from build123d import *

# Parameters (mm, degrees)
SKETCH_1_R          = 25
SKETCH_1_R_2        = 8
SKETCH_1_R_3        = 1.65
EXTRUDE_1_DEPTH     = 4
SKETCH_5_W          = 23.4
SKETCH_5_H          = 29.4
CUT_EXTRUDE_1_DEPTH = 1
SKETCH_6_R          = 3
CUT_EXTRUDE_2_DEPTH = 2.8
CUT_EXTRUDE_3_REACH = 37.482
SKETCH_9_R          = 0.75
CUT_EXTRUDE_START   = -1.1
CUT_EXTRUDE_4_DEPTH = 1.1


with BuildPart() as part:
    # 草图1 → 凸台-拉伸1 (new body)
    with BuildSketch(Plane(origin=(0, 0, 0), x_dir=(1, 0, 0), z_dir=(0, 1, 0))):
        with Locations(Location((0, 0, 0), (0, 0, 270))):
            Circle(SKETCH_1_R)
        with Locations(Location((0, 0, 0), (0, 0, 270))):
            Circle(SKETCH_1_R_2, mode=Mode.SUBTRACT)
        with Locations(Location((10.606601718, 10.606601718, 0), (0, 0, 270))):
            Circle(SKETCH_1_R_3, mode=Mode.SUBTRACT)
        with Locations(Location((-10.606601718, 10.606601718, 0), (0, 0, 270))):
            Circle(SKETCH_1_R_3, mode=Mode.SUBTRACT)
        with Locations(Location((-10.606601718, -10.606601718, 0), (0, 0, 270))):
            Circle(SKETCH_1_R_3, mode=Mode.SUBTRACT)
        with Locations(Location((10.606601718, -10.606601718, 0), (0, 0, 270))):
            Circle(SKETCH_1_R_3, mode=Mode.SUBTRACT)
    extrude(amount=EXTRUDE_1_DEPTH)

    # 草图5 → 切除-拉伸1 (cut)
    with BuildSketch(Plane(origin=(0, 4, 0), x_dir=(1, 0, 0), z_dir=(0, 1, 0))):
        with Locations((0, 6)):
            Rectangle(SKETCH_5_W, SKETCH_5_H)
    extrude(amount=-CUT_EXTRUDE_1_DEPTH, mode=Mode.SUBTRACT)

    # 草图6 → 切除-拉伸2 (cut)
    with BuildSketch(Plane(origin=(0, 4, 0), x_dir=(1, 0, 0), z_dir=(0, 1, 0))):
        with Locations(Location((-10.606601718, 10.606601718, 0), (0, 0, 270))):
            Circle(SKETCH_6_R)
        with Locations(Location((10.606601718, 10.606601718, 0), (0, 0, 270))):
            Circle(SKETCH_6_R)
        with Locations(Location((10.606601718, -10.606601718, 0), (0, 0, 270))):
            Circle(SKETCH_6_R)
        with Locations(Location((-10.606601718, -10.606601718, 0), (0, 0, 270))):
            Circle(SKETCH_6_R)
    extrude(amount=-CUT_EXTRUDE_2_DEPTH, mode=Mode.SUBTRACT)

    # 草图9 → 切除-拉伸3 (cut, up to next)
    with BuildSketch(Plane(origin=(0, 3, 0), x_dir=(1, 0, 0), z_dir=(0, 1, 0)), mode=Mode.PRIVATE) as cut_extrude_3_sk1:
        with Locations(Location((-8.5, 5.5, 0), (0, 0, 270))):
            Circle(SKETCH_9_R)
    cut_extrude_3_tool1 = extrude(cut_extrude_3_sk1.sketch, amount=-CUT_EXTRUDE_3_REACH, mode=Mode.PRIVATE) & part.part
    # 草图9 → 切除-拉伸3 (cut, up to next)
    with BuildSketch(Plane(origin=(0, 3, 0), x_dir=(1, 0, 0), z_dir=(0, 1, 0)), mode=Mode.PRIVATE) as cut_extrude_3_sk2:
        with Locations(Location((8.5, 5.5, 0), (0, 0, 270))):
            Circle(SKETCH_9_R)
    cut_extrude_3_tool2 = extrude(cut_extrude_3_sk2.sketch, amount=-CUT_EXTRUDE_3_REACH, mode=Mode.PRIVATE) & part.part
    # 草图9 → 切除-拉伸3 (cut, up to next)
    with BuildSketch(Plane(origin=(0, 3, 0), x_dir=(1, 0, 0), z_dir=(0, 1, 0)), mode=Mode.PRIVATE) as cut_extrude_3_sk3:
        with Locations(Location((8.5, -5.5, 0), (0, 0, 270))):
            Circle(SKETCH_9_R)
    cut_extrude_3_tool3 = extrude(cut_extrude_3_sk3.sketch, amount=-CUT_EXTRUDE_3_REACH, mode=Mode.PRIVATE) & part.part
    # 草图9 → 切除-拉伸3 (cut, up to next)
    with BuildSketch(Plane(origin=(0, 3, 0), x_dir=(1, 0, 0), z_dir=(0, 1, 0)), mode=Mode.PRIVATE) as cut_extrude_3_sk4:
        with Locations(Location((-8.5, -5.5, 0), (0, 0, 270))):
            Circle(SKETCH_9_R)
    cut_extrude_3_tool4 = extrude(cut_extrude_3_sk4.sketch, amount=-CUT_EXTRUDE_3_REACH, mode=Mode.PRIVATE) & part.part
    add(cut_extrude_3_tool1.solids().sort_by_distance((-8.5, 3, -5.5))[0], mode=Mode.SUBTRACT)
    add(cut_extrude_3_tool2.solids().sort_by_distance((8.5, 3, -5.5))[0], mode=Mode.SUBTRACT)
    add(cut_extrude_3_tool3.solids().sort_by_distance((8.5, 3, 5.5))[0], mode=Mode.SUBTRACT)
    add(cut_extrude_3_tool4.solids().sort_by_distance((-8.5, 3, 5.5))[0], mode=Mode.SUBTRACT)

    # 草图10 → 切除-拉伸4 (cut)
    with BuildSketch(Plane(origin=(0, 3, 0), x_dir=(1, 0, 0), z_dir=(0, 1, 0)).offset(CUT_EXTRUDE_START)):
        with BuildLine():
            Line((-5.700788223, 5.612576381), (-5.700788223, 6.246626792))
            ThreePointArc((-5.700788223, 6.246626792), (-5.993681442, 6.953733574), (-6.700788223, 7.246626792))
            Line((-6.700788223, 7.246626792), (-11.441421376, 7.246626792))
            Line((-11.441421376, 7.246626792), (-11.441421376, 20.219080974))
            Line((-11.441421376, 20.219080974), (11.441421376, 20.219080974))
            Line((11.441421376, 20.219080974), (11.441421376, 7.246626792))
            Line((11.441421376, 7.246626792), (6.700788223, 7.246626792))
            ThreePointArc((6.700788223, 7.246626792), (5.993681442, 6.953733574), (5.700788223, 6.246626792))
            Line((5.700788223, 6.246626792), (5.700788223, 5.612576381))
            ThreePointArc((5.700788223, 5.612576381), (0, 8), (-5.700788223, 5.612576381))
        make_face()
    extrude(amount=CUT_EXTRUDE_4_DEPTH, mode=Mode.SUBTRACT)


solid = part.part
Design review of the part built by this model. Coordinates are the model's own, in mm. A direction names the side the tool comes from. Coordinates: 2 decimals unless noted, no trailing zeros. Order: outer loops, then holes, each group sorted by start corner. A loop starts at its lowest first (then second) coordinate and runs counter-clockwise, first axis right, second up. Notation, with made-up numbers: (10, 19) - (34, 19) arc R18 ccw to (34, 42) - close; hole circle Ø9 at (87, 23). An arc over 180 degrees is marked (long way). Put each result on its own line as item: value.
1) Insertion check: P1, Ø16, axis at x = 2, z = -10.5, coming from the +Y side; P2, Ø1.1, axis at y = 3.5, z = -3, coming from the -X side; P3, Ø3, axis at x = -10.5, z = 9.5, coming from the +Y side. Each pin has a flat end and moves straight along its axis. Give the tip position at first contact, or say it passes through.
Response values:
P1: stops at y = 3
P2: stops at x = -24.88
P3: stops at y = 1.2
2) Take a section at B-B, the plane x = -1. Give the boundary of the cut face in (y, z).
Response values:
outline: (0, -24.98) - (4, -24.98) - (4, -20.7) - (3, -20.7) - (3, -20.22) - (1.9, -20.22) - (1.9, -7.94) - (0, -7.94) - close; (0, 7.94) - (3, 7.94) - (3, 8.7) - (4, 8.7) - (4, 24.98) - (0, 24.98) - close
3) The part is to be moulded in two halves that separate along Z. For faces 1 (the face through (7.509, 1.972, 23.846)), 2 (the face through (0, 1.9, -15)), 3 (the face through (6, 0, -6)), say which applies: released by +Z, released by -Z, zero draft, split by the parting line, or undercut.
Response values:
face 1: split by the parting line
face 2: undercut
face 3: zero draft
4) Take a section at D-D, the plane z = 20. Give the boundary of the cut face in (x, y), and give its area (3 significant figures).
Response values:
outline: (-15, 0) - (15, 0) - (15, 4) - (-15, 4) - close
area: 120 mm²
5) Take a section at A-A, the plane z = 0. Give the boundary of the cut face in (x, y), and give its area (3 significant figures).
Response values:
outline: (-25, 0) - (-8, 0) - (-8, 3) - (-11.7, 3) - (-11.7, 4) - (-25, 4) - close; (8, 0) - (25, 0) - (25, 4) - (11.7, 4) - (11.7, 3) - (8, 3) - close
area: 129 mm²
6) Tool access review of faces 4 (the face through (-0.2, 2.4, -20.219)), 5 (the face through (10.679, 0.592, -12.255)): name each direction out of +Z, -Z, +X, -X, +Y, -Y from which nothing blocks a thin tool from reaching the whole face with its end or side.
Response values:
face 4: +Y
face 5: +Y, -Y
7) Take a section at C-C, the plane z = -11. Give the boundary of the cut face in (x, y), and give its area (3 significant figures).
Response values:
outline: (-22.45, 0) - (-12.21, 0) - (-12.21, 1.2) - (-13.58, 1.2) - (-13.58, 4) - (-22.45, 4) - close; (-9, 0) - (9, 0) - (9, 1.2) - (7.63, 1.2) - (7.63, 1.9) - (-7.63, 1.9) - (-7.63, 1.2) - (-9, 1.2) - close; (12.21, 0) - (22.45, 0) - (22.45, 4) - (13.58, 4) - (13.58, 1.2) - (12.21, 1.2) - close
area: 107 mm²
8) Wall thickness on L1, parallel to X at y = 1.05, z = 0; L2, parallel to Y at x = 6.5, z = 5; L3, parallel to Z at x = 12, y = 1.65: over which ranges is each line inside the solid? List them lowest first. Write a range as from..to.
Response values:
L1: x = -25..-8, 8..25
L2: y = 0..3
L3: z = -21.93..-13.26, -7.95..7.95, 13.26..21.93
